Autodesk Inventor part; units mm, degrees
ref_plane "YZ Plane" through (0, 0, 0) normal (1, 0, 0) x (0, 1, 0)
ref_plane "XZ Plane" through (0, 0, 0) normal (0, 1, 0) x (-1, 0, 0)
ref_plane "XY Plane" through (0, 0, 0) normal (0, 0, 1) x (1, 0, 0)
sketch "Skizze1" plane through (0, 0, 0) normal (1, 0, 0) x (0, 1, 0)
  line L0 (0, 0) -> (115, 0)
  line L1 (115, 0) -> (115, -58.5)
  line L2 (115, -58.5) -> (0, -58.5)
  line L3 (0, -58.5) -> (0, 0)
  line L4 (115, 0) -> (115, -25)
  line L5 (115, -25) -> (100, -25)
  line L6 (100, -25) -> (100, -12.5)
  line L7 (100, -12.5) -> (100, -25)
  line L8 (100, -25) -> (100, -37.5)
  line L9 (100, -25) -> (15, -25)
  line L10 (15, -25) -> (15, -12.5)
  line L11 (15, -12.5) -> (15, -25)
  line L12 (15, -25) -> (15, -37.5)
  circle A0 centre (100, -12.5) radius 3
  circle A1 centre (100, -37.5) radius 3
  circle A2 centre (15, -12.5) radius 3
  circle A3 centre (15, -37.5) radius 3
  line L13 (115, -58.5) -> (85, -58.5)
  line L14 (85, -58.5) -> (50, -58.5)
  line L15 (50, -58.5) -> (10, -58.5)
  line L16 (10, -58.5) -> (10, -53.5)
  line L17 (50, -58.5) -> (50, -53.5)
  line L18 (85, -58.5) -> (85, -53.5)
  circle A4 centre (85, -53.5) radius 2.5
  circle A5 centre (50, -53.5) radius 2.5
  circle A6 centre (10, -53.5) radius 2.5
  dimension "d0" = 115
  dimension "d1" = 58.5
  dimension "d2" = 25
  dimension "d3" = 15
  dimension "d4" = 12.5
  dimension "d5" = 85
  dimension "d6" = 6
  dimension "d7" = 6
  dimension "d8" = 6
  dimension "d9" = 6
  dimension "d10" = 30
  dimension "d11" = 35
  dimension "d12" = 40
  dimension "d13" = 5
  dimension "d14" = 5
  dimension "d15" = 5
  dimension "d16" = 5
  dimension "d17" = 5
  dimension "d18" = 5
extrude "Extrusion1" add sketch "Skizze1" along normal blind 5
properties part number "Motorhalterung_Stützleiste" material "Aluminium 6061"
Geometry: final body of the model. Coordinates: model frame, mm. Give positions to 0.01 mm unless a question says otherwise; leave off trailing zeros. Write each loop counter-clockwise with the first axis right and the second up, starting at its lowest first coordinate (ties: lowest second). Pieces come first, ordered by that corner, then holes.
(1) Cut plane B-B, the plane z = -37.5. Return loops of the section in (x, y).
(2) First-contact query: P1, Ø3.5, axis at y = 100, z = -12.5, coming from the -X side; P2, Ø1, axis at x = 1, z = -13.5, coming from the -Y side. Flat tips, straight axial feed; report the tip coordinate or a pass-through.
(3) Mould query, pull axis Y, two halves, no side actions, for faces 1 (the cylindrical face through (2.46, 97.79, -39.53)), 2 (the cylindrical face through (2.5, 97, -12.6)), 3 (the flat face through (2, 0, -30)), 4 (the flat face through (2, 58, -58.5)). Classes: released by +Y, released by -Y, zero draft, split by the parting line, or undercut.
(4) Cut plane D-D, the plane y = 50. Return loops of the section in (x, z).
(5) Ray query, line 1 (Y direction, x = 2.25, z = -12.5); line 2 (Z direction, x = 2.6, y = 15); line 3 (Y direction, x = 3.8, z = -15). Return the intervals inside material, ascending.
(6) Cut plane A-A, the plane z = -53.5. Return loops of the section in (x, y).
(7) Cut plane C-C, the plane x = 2.7. Return loops of the section in (y, z).
Values follow:
1. outline: (0, 0) - (5, 0) - (5, 12) - (0, 12) - close; (0, 18) - (5, 18) - (5, 97) - (0, 97) - close; (0, 103) - (5, 103) - (5, 115) - (0, 115) - close
2. P1: passes through
2. P2: stops at y = 0
3. face 1: undercut
3. face 2: undercut
3. face 3: released by -Y
3. face 4: zero draft
4. outline: (0, -58.5) - (5, -58.5) - (5, -56) - (0, -56) - close; (0, -51) - (5, -51) - (5, 0) - (0, 0) - close
5. line 1: y = 0 to 12, 18 to 97, 103 to 115
5. line 2: z = -58.5 to -40.5, -34.5 to -15.5, -9.5 to 0
5. line 3: y = 0 to 13.34, 16.66 to 98.34, 101.66 to 115
6. outline: (0, 0) - (5, 0) - (5, 7.5) - (0, 7.5) - close; (0, 12.5) - (5, 12.5) - (5, 47.5) - (0, 47.5) - close; (0, 52.5) - (5, 52.5) - (5, 82.5) - (0, 82.5) - close; (0, 87.5) - (5, 87.5) - (5, 115) - (0, 115) - close
7. outline: (0, -58.5) - (115, -58.5) - (115, 0) - (0, 0) - close; hole circle Ø5 at (10, -53.5); hole circle Ø6 at (15, -37.5); hole circle Ø6 at (15, -12.5); hole circle Ø5 at (50, -53.5); hole circle Ø5 at (85, -53.5); hole circle Ø6 at (100, -37.5); hole circle Ø6 at (100, -12.5)
